Verification items for the finished model (mm, model axes). Give positions to 0.01 mm unless a question says otherwise; leave off trailing zeros. Order: outer loops, then holes, each group sorted by start corner. A loop starts at its lowest first (then second) coordinate and runs counter-clockwise, first axis right, second up. Notation, with made-up numbers: (25, 66) -> (60, 66) arc R16 cw to (60, 92) -> close; hole circle Ø6 at (17.5, 0.25). An arc over 180 degrees is marked (long way). Return JSON: item names as keys, results as strings. Group by question number.
(1) Thickness scan on line 1 along X through (y, z) = (1, -256.54); line 2 along Z through (x, y) = (50.8, 0.25); line 3 along Z through (x, y) = (49, 0.75). Record the ranges inside material, lowest first.
(2) Cross-section at A-A on x = 50.8. Enter the section's corners in (y, z) (1 decimal), then the cut area to 3 significant figures.
(3) Cross-section at C-C on y = 0. Enter the section's corners in (x, z) (1 decimal), then the cut area to 3 significant figures.
(4) Release check for a two-part mould opening along Z. For faces 1 (the face through (150, -3.175, -157)), 2 (the face through (239.726, -0.044, -53.968)) record: pulls with the +Z half, pulls with the -Z half, needs draft (parallel to the pull), parting line crosses it, or undercut.
(5) Depth check by flat-ended pin: pin 1 Ø3 at (y, z) = (-2, -176.5) entering from -X; pin 2 Ø23 at (x, z) = (50.8, -256.54) entering from -Y. Enter the tip coordinate at first touch or a pass-through.
(6) Cross-section at B-B on z = -53.34. Enter the section's corners in (x, y) (1 decimal).
from build123d import *

# Parameters (mm, degrees)
SKETCH1_W           = 304.8
SKETCH1_H           = 309.88
SKETCH1_R           = 14.2875
BOSS_EXTRUDE1_DEPTH = 3.175


with BuildPart() as part:
    # Sketch1 → Boss-Extrude1 (new body, symmetric)
    with BuildSketch(Plane(origin=(0, 0, 0), x_dir=(1, 0, 0), z_dir=(0, 1, 0))):
        with Locations((152.4, 154.94)):
            Rectangle(SKETCH1_W, SKETCH1_H)
        with Locations((50.8, 53.34)):
            Circle(SKETCH1_R, mode=Mode.SUBTRACT)
        with Locations((254, 53.34)):
            Circle(SKETCH1_R, mode=Mode.SUBTRACT)
        with Locations((50.8, 256.54)):
            Circle(SKETCH1_R, mode=Mode.SUBTRACT)
        with Locations((254, 256.54)):
            Circle(SKETCH1_R, mode=Mode.SUBTRACT)
    extrude(amount=BOSS_EXTRUDE1_DEPTH, both=True)


solid = part.part
Verdict:
{
 "1": {"line 1": "0 to 36.51, 65.09 to 239.71, 268.29 to 304.8", "line 2": "-309.88 to -270.83, -242.25 to -67.63, -39.05 to 0", "line 3": "-309.88 to -270.71, -242.37 to -67.51, -39.17 to 0"},
 "2": {"outline": "(-3.2, -309.9) -> (3.2, -309.9) -> (3.2, -270.8) -> (-3.2, -270.8) -> close; (-3.2, -242.3) -> (3.2, -242.3) -> (3.2, -67.6) -> (-3.2, -67.6) -> close; (-3.2, -39.1) -> (3.2, -39.1) -> (3.2, 0) -> (-3.2, 0) -> close", "area": "1,600 mm²"},
 "3": {"outline": "(0, -309.9) -> (304.8, -309.9) -> (304.8, 0) -> (0, 0) -> close; hole circle Ø28.6 at (50.8, -256.5); hole circle Ø28.6 at (50.8, -53.3); hole circle Ø28.6 at (254, -256.5); hole circle Ø28.6 at (254, -53.3)", "area": "91,900 mm²"},
 "4": {"face 1": "needs draft", "face 2": "undercut"},
 "5": {"pin 1": "x = 0", "pin 2": "through"},
 "6": {"outline": "(0, -3.2) -> (36.5, -3.2) -> (36.5, 3.2) -> (0, 3.2) -> close; (65.1, -3.2) -> (239.7, -3.2) -> (239.7, 3.2) -> (65.1, 3.2) -> close; (268.3, -3.2) -> (304.8, -3.2) -> (304.8, 3.2) -> (268.3, 3.2) -> close"}
}
